Could you check a few things on this model? Use its own coordinates, in mm. A direction names the side the tool comes from. Give positions to 0.01 mm unless a question says otherwise; leave off trailing zeros. One line per question, with ' | ' between items.
Autodesk Inventor part; units mm, degrees
ref_plane "YZ Plane" through (0, 0, 0) normal (1, 0, 0) x (0, 1, 0)
ref_plane "XZ Plane" through (0, 0, 0) normal (0, 1, 0) x (-1, 0, 0)
ref_plane "XY Plane" through (0, 0, 0) normal (0, 0, 1) x (1, 0, 0)
sketch "Sketch1" plane through (0, 0, 0) normal (0, 0, 1) x (1, 0, 0)
  circle A0 centre (0, 0) radius 13.2282
  circle A1 centre (0, 0) radius 3.05
  circle A2 centre (-8, 0) radius 1.3525
  circle A3 centre (0, 8) radius 1.3525
  circle A4 centre (8, 0) radius 1.3525
  circle A5 centre (0, -8) radius 1.3525
  dimension "d12" = 6.1
  dimension "d13" = 2.705
  dimension "d14" = 2.705
  dimension "d15" = 2.705
  dimension "d16" = 2.705
extrude "Extrusion1" add sketch "Sketch1" along normal blind 12.7
sketch "Sketch7" plane through (0, 0, 12.7) normal (0, 0, 1) x (1, 0, 0)
  circle A0 centre (0, 0) radius 3.05
  circle A1 centre (0, 0) radius 13.2282
extrude "Extrusion6" add sketch "Sketch7" along normal blind 7.9375
fillet "Fillet2" radius 7.9375 1 edges at (-13.2282, 0, 20.6375)
sketch "Sketch8" plane through (0, 0, 0) normal (0, 0, -1) x (-1, 0, 0)
  circle A0 centre (0, 0) radius 3.175
  dimension "d21" = 6.35
extrude "Extrusion7" cut sketch "Sketch8" against normal through all
chamfer "Chamfer1" distance 1.5875 distance2 3.175 1 edges at (3.175, 0, 20.6375) measured on face at (4.5034, -0.6753, 20.6375)
properties part number "adaptor"
Q1. If I drill on line 1 along Y through (x, z) = (0, 11) (1 decimal); line 2 along Y through (x, z) = (0.75, 4), over which ranges is the centre line in solid material (lowest first)?
Answer below:
line 1: y = -13.2 to -9.4, -6.6 to -3.2, 3.2 to 6.6, 9.4 to 13.2 | line 2: y = -13.21 to -9.13, -6.87 to -3.09, 3.09 to 6.87, 9.13 to 13.21
Q2. If we mould it in two halves opening along X, with no side actions, what happens to faces 3 (the flat face through (3, -3, 0)), 4 (the cylindrical face through (-10.497, 8.049, 6.261)), 5 (the flat face through (0, -8, 12.7))? For each: +X half, -X half, draft (parallel to the pull), parting line (faces both ways), or undercut.
Answer below:
face 3: draft | face 4: parting line | face 5: undercut
Q3. Will these pins go through, and if not, where does the flat tip stop? pin 1 (3.5 mm diameter, centred on x = -8, y = 0, fed in from +Z); pin 2 (4 mm diameter, centred on y = -1.5, z = 6.5, fed in from +X); pin 3 (5.5 mm diameter, centred on x = 0, y = 0, fed in from -Z); pin 4 (2 mm diameter, centred on x = 0, y = -8, fed in from +Z).
Answer below:
pin 1: stops at z = 20.58 | pin 2: stops at x = 13.23 | pin 3: passes through | pin 4: stops at z = 20.45
Q4. On a 3-axis mill with a long thin cutter (end or side, diameter ignored), from which of +Z, -Z, +X, -X, +Y, -Y can I reach the whole of each face in a straight line? I mean faces 1 (the cylindrical face through (0.69, -3.1, 8.61)), 2 (the cylindrical face through (8.62, 1.2, 6.26)). Say none if no direction works.
Answer below:
face 1: +Z, -Z | face 2: -Z
Q5. Imagine slicing it at A-A on z = 5.5. Count the separate pieces of the cut face and the enclosed holes in it, and give its area (3 significant figures).
Answer below:
separate pieces: 1 | enclosed holes: 5 | area: 495 mm^2
